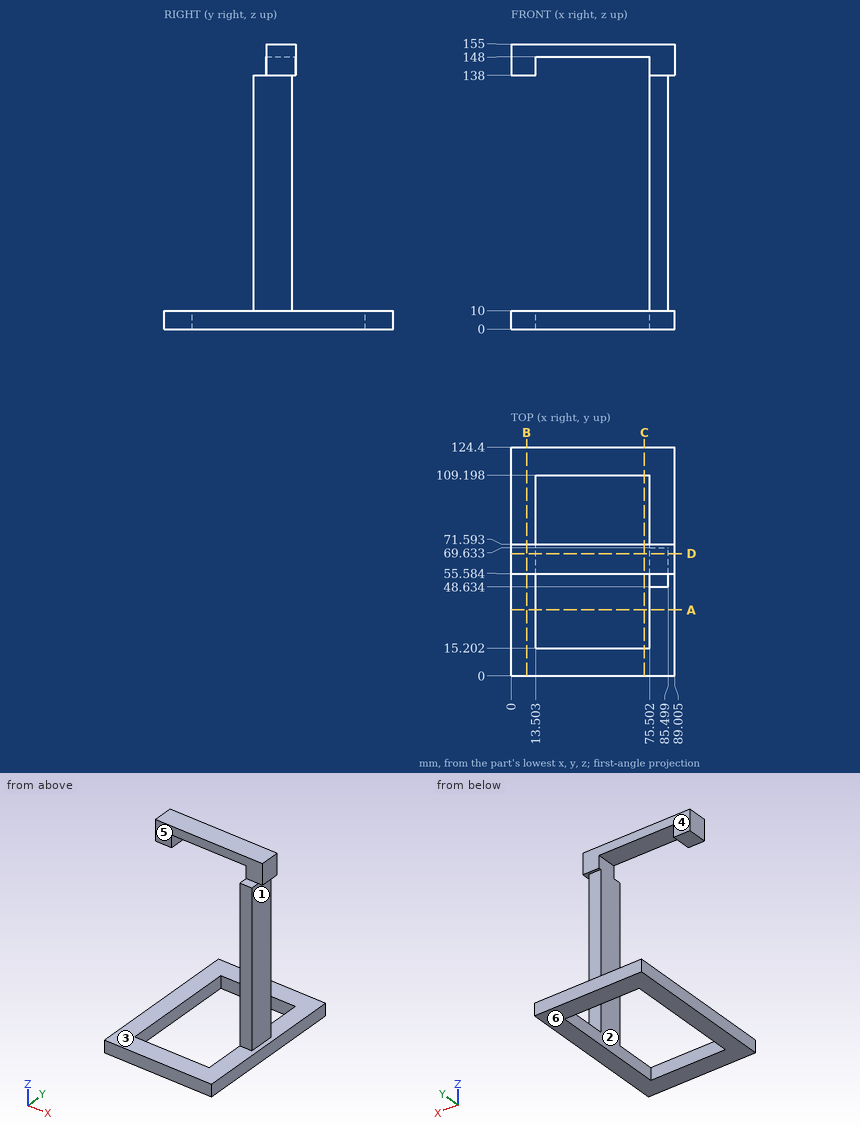
Check sheet for the drawn part. Datum: minimum x, y, z corner. Units: mm. A direction names the side the tool comes from. Round coordinates to 2 decimals unless told otherwise and drop trailing zeros. Order: outer loops, then holes, each group sorted by start corner. A loop starts at its lowest first (then second) coordinate and runs counter-clockwise, first axis right, second up.
(1) Cross-section at D-D, the plane y = 66.5. Enter the section's corners in (x, z) (1 decimal).
(2) Cross-section at A-A, the plane y = 36. Enter the section's corners in (x, z) (1 decimal), and give its area (3 significant figures).
(3) Cross-section at C-C, the plane x = 72.5. Enter the section's corners in (y, z), and give its area (3 significant figures).
(4) Go/stop test with flat-tipped pins: P1, Ø10, axis at x = 19, y = 21.5, coming from the +Z side; P2, Ø3.5, axis at x = 80, y = 52.5, coming from the +Z side; P3, Ø5, axis at x = 79.5, z = 47.5, coming from the -Y side; P4, Ø12, axis at y = 47, z = 106, coming from the +X side. Record where each tip stops, or that it passes through.
(5) Cross-section at B-B, the plane x = 8.5. Enter the section's corners in (y, z), and give its area (3 significant figures).
(6) Scan lines: probe 1 along Z at (x, y) = (8, 65.5); probe 2 along Z at (x, y) = (82.5, 25.5). Record each from-to range of solid material in increasing order.
(7) Access from +Z, -Z, +X, -X, +Y, -Y to the whole of each face (thin tool, end or side, straight path). Record for the marked faces 4, 5 and 6.
(8) Draft check along X on the marked faces 1, 2 and 3. Enter one of: pulls with the +X half, pulls with the -X half, needs draft (parallel to the pull), parting line crosses it, or undercut.
Check sheet entries:
1. outline: (0, 0) - (13.5, 0) - (13.5, 10) - (0, 10) - close; (0, 138) - (13.5, 138) - (13.5, 148) - (75.5, 148) - (75.5, 0) - (89, 0) - (89, 10) - (85.5, 10) - (85.5, 138) - (89, 138) - (89, 155) - (0, 155) - close
2. outline: (0, 0) - (13.5, 0) - (13.5, 10) - (0, 10) - close; (75.5, 0) - (89, 0) - (89, 10) - (75.5, 10) - close
2. area: 270 mm2
3. outline: (0, 0) - (15.2, 0) - (15.2, 10) - (0, 10) - close; (55.58, 148) - (71.59, 148) - (71.59, 155) - (55.58, 155) - close; (109.2, 0) - (124.4, 0) - (124.4, 10) - (109.2, 10) - close
3. area: 416 mm2
4. P1: passes through
4. P2: stops at z = 138
4. P3: stops at y = 48.63
4. P4: stops at x = 85.5
5. outline: (0, 0) - (124.4, 0) - (124.4, 10) - (0, 10) - close; (55.58, 138) - (71.59, 138) - (71.59, 155) - (55.58, 155) - close
5. area: 1,520 mm2
6. probe 1: z = 0 to 10, 138 to 155
6. probe 2: z = 0 to 10
7. face 4: +Z, +X, -X, +Y
7. face 5: +Z, +X, -X, -Y
7. face 6: -Z, +X, -X, +Y, -Y
8. face 1: pulls with the +X half
8. face 2: undercut
8. face 3: needs draft
